Check sheet for the modelled part. Datum: model origin and axes. Units: mm. Face numbers are marked on the shaded views. A direction names the side the tool comes from. Coordinates: 2 decimals unless noted, no trailing zeros. Write each loop counter-clockwise with the first axis right and the second up, starting at its lowest first coordinate (ties: lowest second). Pieces come first, ordered by that corner, then holes. Notation, with made-up numbers: (82.5, -17.75) - (113.5, -17.75) arc R30 ccw to (113.5, 4.25) - close; hole circle Ø3 at (-22, 10). An arc over 180 degrees is marked (long way). Write each question's results on one line, items separated by ' | '.
from build123d import *

# Parameters (mm, degrees)
SKETCH005_R           = 28
SKETCH005_R_2         = 13
PAD002_DEPTH          = 17.5
SKETCH007_R           = 16
POCKET003_DEPTH       = 13.5
SKETCH006_R           = 4
PAD003_DEPTH          = 3
SKETCH008_R           = 1.7
POCKET004_DEPTH       = 17.501
PAD_DEPTH             = 2
POLARPATTERN_COUNT    = 3
CHAMFER_SIZE          = 1
CHAMFER001_SIZE       = 1
CHAMFER002_SIZE       = 1
SKETCH_R              = 3.5
POCKET_DEPTH          = 1.5
POLARPATTERN001_COUNT = 6
CHAMFER003_SIZE       = 1.5
CHAMFER004_SIZE       = 1.5
CHAMFER005_SIZE       = 1.5
CHAMFER006_SIZE       = 1.5
CHAMFER007_SIZE       = 1.5
CHAMFER008_SIZE       = 1.5


with BuildPart() as part:
    # Sketch005 → Pad002 (new body)
    with BuildSketch(Plane.XY):
        Circle(SKETCH005_R)
        Circle(SKETCH005_R_2, mode=Mode.SUBTRACT)
    extrude(amount=PAD002_DEPTH)

    # Sketch007 → Pocket003 (cut)
    with BuildSketch(Plane.XY.offset(17.5)):
        with Locations((0, 22.5)):
            Circle(SKETCH007_R)
        with Locations((-19.485572, -11.25)):
            Circle(SKETCH007_R)
        with Locations((19.485572, -11.25)):
            Circle(SKETCH007_R)
    extrude(amount=-POCKET003_DEPTH, mode=Mode.SUBTRACT)

    # Sketch006 → Pad003 (new body)
    with BuildSketch(Plane.XY.offset(4)):
        with Locations((0, 22.5)):
            Circle(SKETCH006_R)
        with Locations((-19.485572, -11.25)):
            Circle(SKETCH006_R)
        with Locations((19.485572, -11.25)):
            Circle(SKETCH006_R)
    extrude(amount=PAD003_DEPTH)

    # Sketch008 → Pocket004 (cut, through all)
    with BuildSketch(Plane.XY.offset(17.5)):
        with Locations((0, 22.5)):
            Circle(SKETCH008_R)
        with Locations((-19.485572, -11.25)):
            Circle(SKETCH008_R)
        with Locations((19.485572, -11.25)):
            Circle(SKETCH008_R)
        with Locations((-19.485572, 11.25)):
            Circle(SKETCH008_R)
        with Locations((19.485572, 11.25)):
            Circle(SKETCH008_R)
        with Locations((0, -22.5)):
            Circle(SKETCH008_R)
    extrude(amount=-POCKET004_DEPTH, mode=Mode.SUBTRACT)

    # Sketch009 → Pad (new body)
    with BuildSketch(Plane.XY.offset(17.5)):
        with BuildLine():
            Line((-2.25, -12.905328), (-2.25, -17.858821))
            ThreePointArc((-2.25, -17.858821), (0, -18), (2.25, -17.858821))
            Line((2.25, -12.905328), (2.25, -17.858821))
            ThreePointArc((-2.25, -12.905328), (0, -13.1), (2.25, -12.905328))
        make_face()
    pad = extrude(amount=PAD_DEPTH)

    # PolarPattern: Pad ×3 about axis
    polarpattern_axis = Axis((0, 0, 17.5), (0, 0, 1))
    for i in range(1, POLARPATTERN_COUNT):
        add(pad.rotate(polarpattern_axis, i * 360 / POLARPATTERN_COUNT))

    # Chamfer
    chamfer_edges = [part.edges().sort_by_distance(p)[0] for p in [
        (-4, 22.5, 7),
    ]]
    chamfer(chamfer_edges, length=CHAMFER_SIZE)

    # Chamfer001
    chamfer001_edges = [part.edges().sort_by_distance(p)[0] for p in [
        (-23.485572, -11.25, 7),
    ]]
    chamfer(chamfer001_edges, length=CHAMFER001_SIZE)

    # Chamfer002
    chamfer002_edges = [part.edges().sort_by_distance(p)[0] for p in [
        (15.485572, -11.25, 7),
    ]]
    chamfer(chamfer002_edges, length=CHAMFER002_SIZE)

    # Sketch → Pocket (cut)
    with BuildSketch(Plane(origin=(0, 0, 0), x_dir=(1, 0, 0), z_dir=(0, 0, -1))):
        with Locations((0, 22.5)):
            Circle(SKETCH_R)
    pocket = extrude(amount=-POCKET_DEPTH, mode=Mode.SUBTRACT)

    # PolarPattern001: Pocket ×6 about axis
    polarpattern001_axis = Axis((0, 0, 0), (0, 0, -1))
    for i in range(1, POLARPATTERN001_COUNT):
        add(pocket.rotate(polarpattern001_axis, i * 360 / POLARPATTERN001_COUNT), mode=Mode.SUBTRACT)

    # Chamfer003
    chamfer003_edges = [part.edges().sort_by_distance(p)[0] for p in [
        (-1.7, 22.5, 1.5),
    ]]
    chamfer(chamfer003_edges, length=CHAMFER003_SIZE)

    # Chamfer004
    chamfer004_edges = [part.edges().sort_by_distance(p)[0] for p in [
        (-21.185572, 11.25, 1.5),
    ]]
    chamfer(chamfer004_edges, length=CHAMFER004_SIZE)

    # Chamfer005
    chamfer005_edges = [part.edges().sort_by_distance(p)[0] for p in [
        (17.785572, -11.25, 1.5),
    ]]
    chamfer(chamfer005_edges, length=CHAMFER005_SIZE)

    # Chamfer006
    chamfer006_edges = [part.edges().sort_by_distance(p)[0] for p in [
        (17.785572, 11.25, 1.5),
    ]]
    chamfer(chamfer006_edges, length=CHAMFER006_SIZE)

    # Chamfer007
    chamfer007_edges = [part.edges().sort_by_distance(p)[0] for p in [
        (-21.185572, -11.25, 1.5),
    ]]
    chamfer(chamfer007_edges, length=CHAMFER007_SIZE)

    # Chamfer008
    chamfer008_edges = [part.edges().sort_by_distance(p)[0] for p in [
        (-1.7, -22.5, 1.5),
    ]]
    chamfer(chamfer008_edges, length=CHAMFER008_SIZE)


solid = part.part
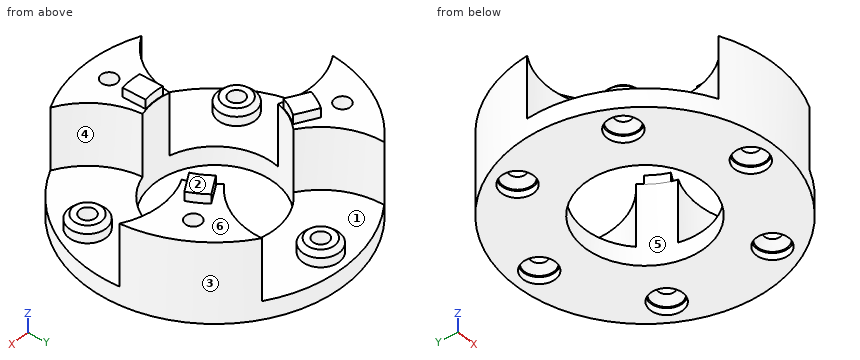
1. Draft check along Y on the marked faces 3, 4, 5 and 6. Enter one of: pulls with the +Y half, pulls with the -Y half, needs draft (parallel to the pull), parting line crosses it, or undercut.
Values follow:
face 3: parting line crosses it | face 4: undercut | face 5: undercut | face 6: needs draft
2. Sectioned sample at C-C (x = 0). Give the number of separate pieces and of enclosed holes in the cut face, then the cut area to 3 significant figures.
Values follow:
separate pieces: 4 | enclosed holes: 0 | area: 257 mm^2
3. Material ranges on L1, parallel to Y at x = 0, z = 0.35; L2, parallel to X at y = 11, z = 14.75; L3, parallel to Z at x = 8.5, y = -13.5, recorded low to high. Write a range as [from, to].
Values follow:
L1: y = [-28, -26], [-19, -13], [13, 19], [26, 28] | L2: x = [-25.75, -21.17], [-17.8, -11.12], [11.12, 17.8], [21.17, 25.75] | L3: z = [0, 4]
4. Access from +Z, -Z, +X, -X, +Y, -Y to the whole of each face (thin tool, end or side, straight path). Record for the marked faces 1 and 2.
Values follow:
face 1: +Z | face 2: +Z, +X, -X, +Y, -Y
5. Go/stop test with flat-tipped pins: pin 1 (1.5 mm diameter, centred on y = -13, z = 2.5, fed in from -X); pin 2 (4 mm diameter, centred on x = 19.49, y = -11.25, fed in from -Z); pin 3 (5.5 mm diameter, centred on x = 19.49, y = -11.25, fed in from -Z). Record where each tip stops, or that it passes through.
Values follow:
pin 1: stops at x = -25.18 | pin 2: stops at z = 2.7 | pin 3: stops at z = 1.95
6. Sectioned sample at A-A (y = 0). Record the cut outline in (x, z), then the cut area to 3 significant figures.
Values follow:
outline: (-28, 0) - (-13, 0) - (-13, 4) - (-28, 4) - close; (13, 0) - (28, 0) - (28, 4) - (13, 4) - close | area: 120 mm^2
7. Sectioned sample at B-B (z = 11.5). Record the cut outline in (x, y), then the cut area to 3 significant figures.
Values follow:
outline: (-27.9, 2.36) arc R16 cw to (-12.6, 3.19) arc R13 cw to (-9.07, 9.32) arc R16 cw to (-15.99, 22.98) arc R28 ccw to start; (-11.91, -25.34) arc R28 ccw to (11.91, -25.34) arc R16 cw to (3.54, -12.51) arc R13 cw to (-3.54, -12.51) arc R16 cw to start; (9.07, 9.32) arc R13 cw to (12.6, 3.19) arc R16 cw to (27.9, 2.36) arc R28 ccw to (15.99, 22.98) arc R16 cw to start; hole circle Ø3.4 at (-19.49, 11.25); hole circle Ø3.4 at (0, -22.5); hole circle Ø3.4 at (19.49, 11.25) | area: 567 mm^2
